The listing builds one solid part. Answer for the finished solid, in the listing's coordinates (mm). A direction names the side the tool comes from. Coordinates: 2 decimals unless noted, no trailing zeros. Answer as CSV lines item,"result". Start each with the question number.
```python
from build123d import *

# Parameters (mm, degrees)
SKETCH1_R      = 3.4
EXTRUDE1_DEPTH = 300


with BuildPart() as part:
    # Sketch1 → Extrude1 (new body)
    with BuildSketch(Plane.XY):
        with BuildLine():
            Line((16.824999974, 19.999999706), (5.628698889, 19.999999706))
            ThreePointArc((5.628698889, 19.999999706), (4.46721611, 19.488662348), (4.059999948, 18.286712625))
            Line((4.059999948, 18.286712625), (4.059999948, 17.5148))
            ThreePointArc((4.059999948, 17.5148), (4.521248189, 16.401248241), (5.634799948, 15.94))
            Line((5.634799948, 15.94), (6.872423693, 15.94))
            Line((6.872423693, 15.94), (6.899033319, 16.702000002))
            Line((6.899033319, 16.702000002), (9.014999977, 16.702000002))
            ThreePointArc((9.014999977, 16.702000002), (9.913025591, 16.330025613), (10.28499998, 15.431999998))
            Line((10.28499998, 15.431999998), (10.28499998, 14.064318961))
            ThreePointArc((10.28499998, 14.064318961), (10.217328883, 13.724113383), (10.024617903, 13.435701022))
            Line((10.024617903, 13.435701022), (5.665101027, 9.076184193))
            ThreePointArc((5.665101027, 9.076184193), (4.124155011, 8.046556992), (2.306485256, 7.685))
            Line((2.306485256, 7.685), (-2.306485308, 7.685))
            ThreePointArc((-2.306485308, 7.685), (-4.124155063, 8.046556992), (-5.665101079, 9.076184193))
            Line((-5.665101079, 9.076184193), (-10.024617955, 13.435701022))
            ThreePointArc((-10.024617955, 13.435701022), (-10.217328935, 13.724113383), (-10.285000032, 14.064318961))
            Line((-10.285000032, 14.064318961), (-10.285000032, 15.431999998))
            ThreePointArc((-10.285000032, 15.431999998), (-9.913025643, 16.330025613), (-9.015000029, 16.702000002))
            Line((-9.015000029, 16.702000002), (-6.899033371, 16.702000002))
            Line((-6.899033371, 16.702000002), (-6.872423745, 15.94))
            Line((-6.872423745, 15.94), (-5.6348, 15.94))
            ThreePointArc((-5.6348, 15.94), (-4.521248241, 16.401248241), (-4.06, 17.5148))
            Line((-4.06, 17.5148), (-4.06, 18.286712625))
            ThreePointArc((-4.06, 18.286712625), (-4.467216162, 19.488662348), (-5.628698941, 19.999999706))
            Line((-5.628698941, 19.999999706), (-16.825000026, 19.999999706))
            ThreePointArc((-16.825000026, 19.999999706), (-19.070064069, 19.070063731), (-20.000000044, 16.824999688))
            Line((-20.000000044, 16.824999688), (-20.000000044, -16.825000312))
            ThreePointArc((-20.000000044, -16.825000312), (-19.070064069, -19.070064355), (-16.825000026, -20.00000033))
            Line((-16.825000026, -20.00000033), (16.824999974, -20.00000033))
            ThreePointArc((16.824999974, -20.00000033), (19.070064017, -19.070064355), (19.999999992, -16.825000312))
            Line((19.999999992, -16.825000312), (19.999999992, 16.824999688))
            ThreePointArc((19.999999992, 16.824999688), (19.070064017, 19.070063731), (16.824999974, 19.999999706))
        make_face()
        Circle(SKETCH1_R, mode=Mode.SUBTRACT)
        with BuildLine():
            Line((-7.685000123, -2.306485221), (-7.685000123, 2.306485342))
            ThreePointArc((-7.685000123, 2.306485342), (-8.046557115, 4.124155098), (-9.076184316, 5.665101114))
            Line((-9.076184316, 5.665101114), (-11.032179452, 7.621096271))
            ThreePointArc((-11.032179452, 7.621096271), (-11.720432933, 8.651140405), (-11.962115415, 9.866160302))
            Line((-11.962115415, 9.866160302), (-11.962115415, 18.508608264))
            ThreePointArc((-11.962115415, 18.508608264), (-12.073707729, 18.778015942), (-12.343115407, 18.889608256))
            Line((-12.343115407, 18.889608256), (-15.556000031, 18.889608256))
            ThreePointArc((-15.556000031, 18.889608256), (-17.53165638, 18.071264601), (-18.350000035, 16.095608252))
            Line((-18.350000035, 16.095608252), (-18.350000035, -15.374719595))
            ThreePointArc((-18.350000035, -15.374719595), (-18.185883968, -15.620336647), (-17.8961589, -15.562706749))
            Line((-17.8961589, -15.562706749), (-11.992569935, -9.659117847))
            ThreePointArc((-11.992569935, -9.659117847), (-11.827389014, -9.411907131), (-11.769385188, -9.120302208))
            Line((-11.769385188, -9.120302208), (-11.769385188, -8.67393273))
            ThreePointArc((-11.769385188, -8.67393273), (-11.711381362, -8.382327807), (-11.546200441, -8.135117091))
            Line((-11.546200441, -8.135117091), (-9.076184352, -5.665101029))
            ThreePointArc((-9.076184352, -5.665101029), (-8.046557124, -4.124155), (-7.685000123, -2.306485221))
        make_face(mode=Mode.SUBTRACT)
        with BuildLine():
            Line((11.769385136, -8.67393273), (11.769385136, -9.120302208))
            ThreePointArc((11.769385136, -9.120302208), (11.827388962, -9.411907131), (11.992569883, -9.659117847))
            Line((11.992569883, -9.659117847), (17.896158848, -15.562706749))
            ThreePointArc((17.896158848, -15.562706749), (18.185883916, -15.620336647), (18.349999983, -15.374719595))
            Line((18.349999983, -15.374719595), (18.349999983, 16.095608252))
            ThreePointArc((18.349999983, 16.095608252), (17.531656328, 18.071264601), (15.555999979, 18.889608256))
            Line((15.555999979, 18.889608256), (12.343115355, 18.889608256))
            ThreePointArc((12.343115355, 18.889608256), (12.073707677, 18.778015942), (11.962115363, 18.508608264))
            Line((11.962115363, 18.508608264), (11.962115363, 9.866160302))
            ThreePointArc((11.962115363, 9.866160302), (11.720432881, 8.651140405), (11.0321794, 7.621096271))
            Line((11.0321794, 7.621096271), (9.076184264, 5.665101114))
            ThreePointArc((9.076184264, 5.665101114), (8.046557063, 4.124155098), (7.685000071, 2.306485342))
            Line((7.685000071, 2.306485342), (7.685000071, -2.306485221))
            ThreePointArc((7.685000071, -2.306485221), (8.046557072, -4.124155), (9.0761843, -5.665101029))
            Line((9.0761843, -5.665101029), (11.546200389, -8.135117091))
            ThreePointArc((11.546200389, -8.135117091), (11.71138131, -8.382327807), (11.769385136, -8.67393273))
        make_face(mode=Mode.SUBTRACT)
        with BuildLine():
            Line((15.588203795, -17.921655982), (9.729110898, -12.062563022))
            ThreePointArc((9.729110898, -12.062563022), (9.481900182, -11.897382101), (9.190295259, -11.839378275))
            Line((9.190295259, -11.839378275), (8.743925781, -11.839378275))
            ThreePointArc((8.743925781, -11.839378275), (8.452320858, -11.781374449), (8.205110142, -11.616193528))
            Line((8.205110142, -11.616193528), (5.665101063, -9.076184423))
            ThreePointArc((5.665101063, -9.076184423), (4.124155035, -8.046557195), (2.306485256, -7.685000194))
            Line((2.306485256, -7.685000194), (-2.306485308, -7.685000194))
            ThreePointArc((-2.306485308, -7.685000194), (-4.124155087, -8.046557195), (-5.665101115, -9.076184423))
            Line((-5.665101115, -9.076184423), (-8.205110194, -11.616193528))
            ThreePointArc((-8.205110194, -11.616193528), (-8.45232091, -11.781374449), (-8.743925833, -11.839378275))
            Line((-8.743925833, -11.839378275), (-9.190295311, -11.839378275))
            ThreePointArc((-9.190295311, -11.839378275), (-9.481900233, -11.897382101), (-9.72911095, -12.062563022))
            Line((-9.72911095, -12.062563022), (-15.588203847, -17.921655982))
            ThreePointArc((-15.588203847, -17.921655982), (-15.64259606, -18.195104108), (-15.410777932, -18.350000028))
            Line((-15.410777932, -18.350000028), (15.41077788, -18.350000028))
            ThreePointArc((15.41077788, -18.350000028), (15.642596008, -18.195104108), (15.588203795, -17.921655982))
        make_face(mode=Mode.SUBTRACT)
    extrude(amount=-EXTRUDE1_DEPTH)


solid = part.part
```
Item 1: For a pull along X with two mould halves and no side action, classify faces 4 (the face through (-11.962, 14, -148)), 5 (the face through (-2, -4, 0)), 6 (the face through (20, 0, -148)), 7 (the face through (-20, 0, -148)) as pulls with the +X half, pulls with the -X half, needs draft (parallel to the pull), parting line crosses it, or undercut.
Item 2: Each of these flat-tipped pins is pushed along its axis until it touches: P1, Ø10, axis at x = 0, z = -196, coming from the +Y side; P2, Ø5, axis at x = -1, z = -98, coming from the +Y side. Where does it stop, or does it pass through?
Item 3: Section A-A on z = -30 is taken. State how many separate pieces and enclosed holes the cut face has, then the cut area to 3 significant figures.
Item 4: For faces 1 (the face through (11, 20, -148)), 2 (the face through (0, 7.685, -148)), 3 (the face through (7.685, 0, -148)), determine the directions among +Z, -Z, +X, -X, +Y, -Y from which every point of the face is accessible in a straight line to the end or side of a thin tool.
Item 5: Consider line 1 (Y direction, x = 0, z = -66.5) (3 decimals); line 2 (X direction, y = -13.5, z = -198.5); line 3 (X direction, y = -6, z = -177). Determine where each line is inside the solid, lowest interval first.
Results are:
1,face 4,"undercut"
1,face 5,"needs draft"
1,face 6,"pulls with the +X half"
1,face 7,"pulls with the -X half"
2,P1,"y = 19.87"
2,P2,"y = 7.84"
3,separate pieces,"1"
3,enclosed holes,"4"
3,area,"655 mm²"
4,face 1,"+Z, -Z, +X, -X, +Y"
4,face 2,"+Z, -Z, +Y"
4,face 3,"+Z, -Z"
5,line 1,"-20 to -18.35, -7.685 to -3.4, 3.4 to 7.685"
5,line 2,"-20 to -18.35, -15.83 to -11.17, 11.17 to 15.83, 18.35 to 20"
5,line 3,"-20 to -18.35, -9.41 to 9.41, 18.35 to 20"
